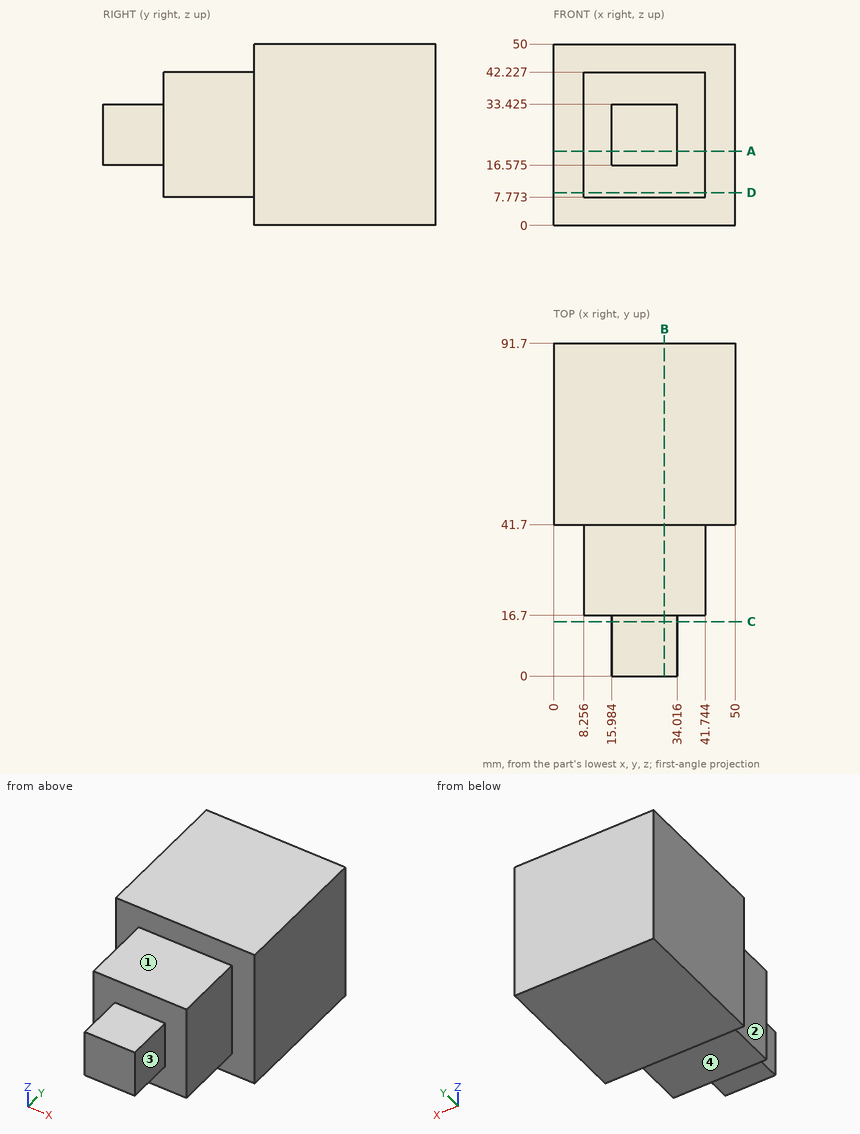
Geometry check sheet. Reference: drawing and pictorial views, mm from the part's lowest x, y, z. A direction names the side the tool comes from. Round coordinates to 2 decimals unless told otherwise and drop trailing zeros. Order: outer loops, then holes, each group sorted by start corner. A loop starts at its lowest first (then second) coordinate and runs counter-clockwise, first axis right, second up. Notation, with made-up numbers: M 76.25,11.25 L 83.25,11.25 A14 cw 83.25,20.25 Z; hole C 74,2 d11. An arc over 180 degrees is marked long. Answer as CSV lines item,"result".
1) Tool access check on the marked faces 1, 2, 3 and 4. Record the directions out of +Z, -Z, +X, -X, +Y, -Y that give a thin tool (end or side, any length) a straight path to the whole face; none if there is none.
Entries:
face 1,"+Z, +X, -X, -Y"
face 2,"+Z, -Z, -X, -Y"
face 3,"+Z, -Z, +X, -Y"
face 4,"-Z, +X, -X, -Y"
2) Sectioned sample at D-D on z = 9. Record the cut outline in (x, y), and give its area (3 significant figures).
Entries:
outline,"M 0,41.7 L 8.26,41.7 L 8.26,16.7 L 41.74,16.7 L 41.74,41.7 L 50,41.7 L 50,91.7 L 0,91.7 Z"
area,"3,340 mm2"
3) Sectioned sample at A-A on z = 20.5. Record the cut outline in (x, y) (1 decimal).
Entries:
outline,"M 0,41.7 L 8.3,41.7 L 8.3,16.7 L 16,16.7 L 16,0 L 34,0 L 34,16.7 L 41.7,16.7 L 41.7,41.7 L 50,41.7 L 50,91.7 L 0,91.7 Z"
4) Sectioned sample at C-C on y = 15. Record the cut outline in (x, z) (1 decimal), and give its area (3 significant figures).
Entries:
outline,"M 16,16.6 L 34,16.6 L 34,33.4 L 16,33.4 Z"
area,"304 mm2"
5) Sectioned sample at B-B on x = 30.5. Record the cut outline in (y, z) (1 decimal).
Entries:
outline,"M 0,16.6 L 16.7,16.6 L 16.7,7.8 L 41.7,7.8 L 41.7,0 L 91.7,0 L 91.7,50 L 41.7,50 L 41.7,42.2 L 16.7,42.2 L 16.7,33.4 L 0,33.4 Z"
6) Thickness scan on probe 1 along Y at (x, z) = (10, 30); probe 2 along X at (y, z) = (18, 26.5); probe 3 along Z at (x, y) = (39, 29.5). Record the ranges inside material, lowest first. Write a range as [from, to].
Entries:
probe 1,"[16.7, 91.7]"
probe 2,"[8.26, 41.74]"
probe 3,"[7.77, 42.23]"
7) Gauge pin test, flat ends, axial feed: pin 1 Ø12.5 at (y, z) = (31, 17.5) entering from +X; pin 2 Ø3 at (x, z) = (23, 14.5) entering from -Y; pin 3 Ø2 at (x, y) = (38.5, 19.5) entering from -Z. Record the tip position at first contact, or that the pin passes through.
Entries:
pin 1,"x = 41.74"
pin 2,"y = 16.7"
pin 3,"z = 7.77"
